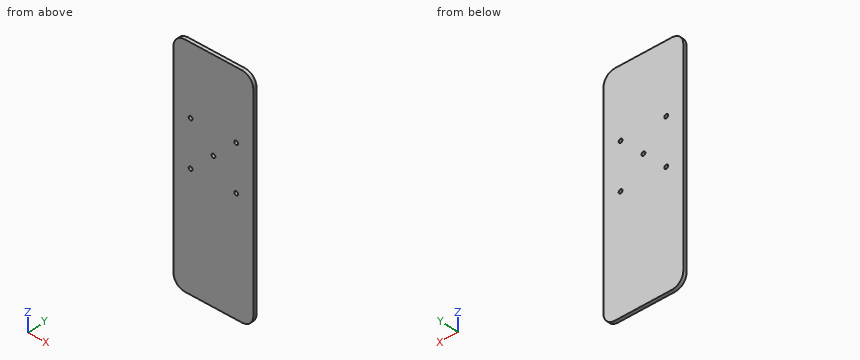
from build123d import *

# Parameters (mm, degrees)
SALIENTE_EXTRUIR1_DEPTH      = 3
TALADRO_DE_MARGEN_PARA_M31_D = 3.4


with BuildPart() as part:
    # Croquis1 → Saliente-Extruir1 (new body)
    with BuildSketch(Plane(origin=(0, 0, 0), x_dir=(1, 0, 0), z_dir=(0, 1, 0))):
        with BuildLine():
            Line((-25, -100), (25, -100))
            ThreePointArc((25, -100), (32.071067812, -97.071067812), (35, -90))
            Line((35, -90), (35, 90))
            ThreePointArc((35, 90), (32.071067812, 97.071067812), (25, 100))
            Line((25, 100), (-25, 100))
            ThreePointArc((-25, 100), (-32.071067812, 97.071067812), (-35, 90))
            Line((-35, 90), (-35, -90))
            ThreePointArc((-35, -90), (-32.071067812, -97.071067812), (-25, -100))
        make_face()
    extrude(amount=SALIENTE_EXTRUIR1_DEPTH)

    # Taladro de margen para M31 (through all)
    with Locations(Plane(origin=(0, 3, 0), x_dir=(1, 0, 0), z_dir=(0, 1, 0))):
        with Locations((-20, 0), (-20, -40), (20, -40), (20, 0), (0, -20)):
            Hole(TALADRO_DE_MARGEN_PARA_M31_D / 2)


solid = part.part
Part model, mm, in its own coordinate system. Coordinates: 2 decimals unless noted, no trailing zeros. Order: outer loops, then holes, each group sorted by start corner. A loop starts at its lowest first (then second) coordinate and runs counter-clockwise, first axis right, second up. Notation, with made-up numbers: M -8.75,-4.75 L 17.25,-4.75 A18 ccw 17.25,15.25 Z; hole C 17,46.25 d4. An arc over 180 degrees is marked long. Use a Markdown table: item, result.
(1) Cut at D-D on x = 0. Write the cut outline in (y, z), then the cut area to 3 significant figures.
A:
| item | result |
|---|---|
| outline | M 0,-100 L 3,-100 L 3,18.3 L 0,18.3 Z; M 0,21.7 L 3,21.7 L 3,100 L 0,100 Z |
| area | 590 mm^2 |
(2) Cut at B-B on x = -20. Write the cut outline in (y, z), then the cut area to 3 significant figures.
A:
| item | result |
|---|---|
| outline | M 0,-100 L 3,-100 L 3,-1.7 L 0,-1.7 Z; M 0,1.7 L 3,1.7 L 3,38.3 L 0,38.3 Z; M 0,41.7 L 3,41.7 L 3,100 L 0,100 Z |
| area | 580 mm^2 |
(3) Probe L1, parallel to Z at x = -20, y = 2.2; L2, parallel to X at y = 0.9, z = 40; L3, parallel to X at y = 2.05, z = 39. List the from-to ranges inside material, lowest first.
A:
| item | result |
|---|---|
| L1 | z = -100 to -1.7, 1.7 to 38.3, 41.7 to 100 |
| L2 | x = -35 to -21.7, -18.3 to 18.3, 21.7 to 35 |
| L3 | x = -35 to -21.37, -18.63 to 18.63, 21.37 to 35 |
(4) Cut at C-C on z = 20. Write the cut outline in (x, y), then the cut area to 3 significant figures.
A:
| item | result |
|---|---|
| outline | M -35,0 L -1.7,0 L -1.7,3 L -35,3 Z; M 1.7,0 L 35,0 L 35,3 L 1.7,3 Z |
| area | 200 mm^2 |
(5) Cut at A-A on z = 40. Write the cut outline in (x, y).
A:
| item | result |
|---|---|
| outline | M -35,0 L -21.7,0 L -21.7,3 L -35,3 Z; M -18.3,0 L 18.3,0 L 18.3,3 L -18.3,3 Z; M 21.7,0 L 35,0 L 35,3 L 21.7,3 Z |
